from build123d import *

# Parameters (mm, degrees)
BOSS_EXTRU_1_DEPTH                               = 63.5
CHANFREIN1_SIZE                                  = 23.8125
CHANFREIN1_SIZE2                                 = 13.748153285
ENL_V_MAT_EXTRU_1_DEPTH                          = 19.05
CHAMBRAGE_POUR_VIS_T_TE_RONDE_BOMB_E_D           = 12.7
CHAMBRAGE_POUR_VIS_T_TE_RONDE_BOMB_E_CBORE_D     = 19.05
CHAMBRAGE_POUR_VIS_T_TE_RONDE_BOMB_E_CBORE_DEPTH = 9.525
ENL_V_MAT_EXTRU_2_DEPTH                          = 4.7625


with BuildPart() as part:
    # Esquisse1 → Boss.-Extru.1 (new body)
    with BuildSketch(Plane.XY):
        Polygon((0, 0), (31.75, 0), (31.75, -4.7625), (50.8, -4.7625), (50.8, 0), (82.55, 0), (82.55, 34.925), (0, 34.925), align=None)
    extrude(amount=BOSS_EXTRU_1_DEPTH)

    # Chanfrein1
    chanfrein1_edges = [part.edges().sort_by_distance(p)[0] for p in [
        (41.275, 34.925, 0),
    ]]
    chanfrein1_side = [part.faces().sort_by_distance(p)[0] for p in [
        (41.275, 34.925, 31.75),
    ]]
    chamfer(chanfrein1_edges, length=CHANFREIN1_SIZE, length2=CHANFREIN1_SIZE2, reference=chanfrein1_side[0])

    # Esquisse2 → Enlèv. mat.-Extru.1 (cut)
    with BuildSketch(Plane(origin=(0, 34.925, 0), x_dir=(1, 0, 0), z_dir=(0, 1, 0))):
        Polygon((50.8, 0), (50.8, -10.526552809), (6.35, -63.5), (82.55, -63.5), (82.55, 0), align=None)
    extrude(amount=-ENL_V_MAT_EXTRU_1_DEPTH, mode=Mode.SUBTRACT)

    # Chambrage pour vis à tête ronde bombée #01 (through all)
    with Locations(Plane(origin=(0, 15.875, 0), x_dir=(1, 0, 0), z_dir=(0, 1, 0))):
        with Locations((41.275, -44.45)):
            CounterBoreHole(CHAMBRAGE_POUR_VIS_T_TE_RONDE_BOMB_E_D / 2, CHAMBRAGE_POUR_VIS_T_TE_RONDE_BOMB_E_CBORE_D / 2, CHAMBRAGE_POUR_VIS_T_TE_RONDE_BOMB_E_CBORE_DEPTH)

    # Esquisse5 → Enlèv. mat.-Extru.2 (cut)
    with BuildSketch(Plane(origin=(0, 15.875, 0), x_dir=(1, 0, 0), z_dir=(0, 1, 0))):
        Polygon((57.15, -63.5), (82.55, -63.5), (82.55, -33.229458748), align=None)
    extrude(amount=-ENL_V_MAT_EXTRU_2_DEPTH, mode=Mode.SUBTRACT)


solid = part.part
The listing builds one solid part. Answer for the finished solid, in the listing's coordinates (mm). A direction names the side the tool comes from. Give positions to 0.01 mm unless a question says otherwise; leave off trailing zeros. Order: outer loops, then holes, each group sorted by start corner. A loop starts at its lowest first (then second) coordinate and runs counter-clockwise, first axis right, second up. Notation, with made-up numbers: (37, -22.5) -> (77, -22.5) arc R30 cw to (77, 16.5) -> close; hole circle Ø10 at (36, 68). An arc over 180 degrees is marked (long way). Put each result on its own line as item: value.
Item 1: Given P1, Ø16, axis at x = 65.5, z = 41, coming from the -Y side; P2, Ø4, axis at x = 58, y = 9, coming from the -Z side; P3, Ø7.5, axis at x = 75, z = 51, coming from the +Y side; P4, Ø11.5, axis at x = 41.275, z = 44.45, coming from the -Y side, each flat-ended and moving along its own axis, determine where each tip first touches the part or whether it passes through.
Established:
P1: stops at y = 0
P2: stops at z = 0
P3: stops at y = 11.11
P4: passes through
Item 2: For a pull along Z with two mould halves and no side action, classify faces 5 (the face through (47.5, 6.35, 46.4)), 6 (the face through (16, 0, 31)), 7 (the face through (70.03, 13.53, 48.15)) as released by +Z, released by -Z, zero draft, split by the parting line, or undercut.
Established:
face 5: undercut
face 6: zero draft
face 7: released by +Z
Item 3: A cutting plane is placed at A-A on y = 4. Give the vertices of the cut face in (x, z) (3 decimals).
Established:
outline: (0, 0) -> (82.55, 0) -> (82.55, 63.5) -> (0, 63.5) -> close; hole circle Ø12.7 at (41.275, 44.45)
Item 4: For faces 1 (the face through (66, 0, 31)), 2 (the face through (50.8, 20, 6)), 3 (the face through (31.75, -2, 31)), 4 (the face through (52, 15.875, 31)), determine the directions among +Z, -Z, +X, -X, +Y, -Y from which every point of the face is accessible in a straight line to the end or side of a thin tool.
Established:
face 1: +Z, -Z, +X, -Y
face 2: +Z, -Z, +X, +Y
face 3: +Z, -Z, -X, -Y
face 4: +Z, +X, +Y
Item 5: A cutting plane is placed at D-D on y = 17. Give the vertices of the cut face in (x, z), plus the area to 3 significant figures.
Established:
outline: (0, 0) -> (50.8, 0) -> (50.8, 10.53) -> (6.35, 63.5) -> (0, 63.5) -> close
area: 2,050 mm^2
Item 6: Straight lines are drawn through the part: line 1 (X direction, y = 1.5, z = 44.45) (3 decimals); line 2 (X direction, y = 9, z = 44); line 3 (Y direction, x = 61.5, z = 60.5). For each, find the intervals that lie inside material, in ascending order.
Established:
line 1: x = 0 to 34.925, 47.625 to 82.55
line 2: x = 0 to 31.76, 50.79 to 82.55
line 3: y = 0 to 11.11
